Read the model definition and answer for the solid it produces. Units are mm, in the model's axes. Face numbers are marked on the shaded views. A direction names the side the tool comes from. Coordinates: 2 decimals unless noted, no trailing zeros. Write each loop counter-clockwise with the first axis right and the second up, starting at its lowest first coordinate (ties: lowest second). Pieces come first, ordered by that corner, then holes. Notation, with made-up numbers: (87, 68.25) -> (137, 68.25) arc R35 cw to (137, 103.25) -> close; hole circle Ø1 at (52.5, -21). An arc over 180 degrees is marked (long way). Answer in a Markdown table with one row per item. Add a question column.
Item 1: Section B-B on z = 0 is taken. Count the separate pieces of the cut face and the enclosed holes in it, then the cut area to 3 significant figures.
Item 2: Given pin 1 Ø6.5 at (y, z) = (-17.25, 0) entering from -X; pin 2 Ø5 at (x, y) = (-9, 2) entering from -Z; pin 3 Ø4 at (x, y) = (-1.5, -28) entering from +Z, each flat-ended and moving along its own axis, determine where each tip first touches the part or whether it passes through.
Item 3: For a pull along Y with two mould halves and no side action, classify the marked faces 3, 4 and 5 as +Y half, -Y half, draft (parallel to the pull), parting line (faces both ways), or undercut.
Item 4: Straight lines are drawn through the part: line 1 (Y direction, x = 1.5, z = 0); line 2 (Z direction, x = 8.5, y = -9); line 3 (X direction, y = 18, z = -2). For each, find the intervals that lie inside material, in ascending order. Write a range as from..to.
Item 5: Which of the six approach directions +Z, -Z, +X, -X, +Y, -Y give full straight-line access (tool end or side, diameter ignored) to the marked faces 1 and 2?
Item 6: Section A-A on x = 2.5 is taken. Write down the section's boundary in (y, z) (3 decimals).
```python
from build123d import *

# Parameters (mm, degrees)
SKETCH_1_R         = 28.5
SKETCH_1_R_2       = 1.9
SKETCH_1_R_3       = 7.5
EXTRUDE_1_DEPTH    = 10
SKETCH3_R          = 1.9
SKETCH3_R_2        = 7.5
CUT_EXTRUDE1_DEPTH = 60.270566179
SKETCH4_R          = 4
CUT_EXTRUDE2_DEPTH = 5


with BuildPart() as part:
    # 草图1 → 凸台-拉伸1 (new body)
    with BuildSketch(Plane(origin=(0, 0, 0), x_dir=(0, 0, -1), z_dir=(1, 0, 0))):
        Circle(SKETCH_1_R)
        with Locations((0, 17.25)):
            Circle(SKETCH_1_R_2, mode=Mode.SUBTRACT)
        with Locations((14.938938215, 8.625)):
            Circle(SKETCH_1_R_2, mode=Mode.SUBTRACT)
        with Locations((14.938938215, -8.625)):
            Circle(SKETCH_1_R_2, mode=Mode.SUBTRACT)
        with Locations((0, -17.25)):
            Circle(SKETCH_1_R_2, mode=Mode.SUBTRACT)
        with Locations((-14.938938215, -8.625)):
            Circle(SKETCH_1_R_2, mode=Mode.SUBTRACT)
        with Locations((-14.938938215, 8.625)):
            Circle(SKETCH_1_R_2, mode=Mode.SUBTRACT)
        Circle(SKETCH_1_R_3, mode=Mode.SUBTRACT)
    extrude(amount=EXTRUDE_1_DEPTH)

    # Sketch2 → Revolve1 (revolve)
    with BuildSketch(Plane.XY):
        with BuildLine():
            Line((0, 0), (-15, 0))
            Line((-15, 0), (-15, 38))
            Line((-15, 38), (-13, 38))
            add(Edge.make_bspline(
                [(-13, 38), (-9.977066976, 32.039576737), (-7.515495422, 32.019303811), (-5.003056497, 32.052880233), (-2, 38)],
                knots=[0.048051887, 0.048051887, 0.048051887, 0.048051887, 0.500504931, 0.951948113, 0.951948113, 0.951948113, 0.951948113], degree=3))
            Line((-2, 38), (0, 38))
            Line((0, 38), (0, 0))
        make_face()
    revolve(axis=Axis((0, 0, 0), (-1, 0, 0)))

    # Sketch3 → Cut-Extrude1 (cut, through all)
    with BuildSketch(Plane(origin=(10, 0, 0), x_dir=(0, 0, -1), z_dir=(1, 0, 0))):
        with Locations((14.938938215, 8.625)):
            Circle(SKETCH3_R)
        with Locations((14.938938215, -8.625)):
            Circle(SKETCH3_R)
        with Locations((0, -17.25)):
            Circle(SKETCH3_R)
        with Locations((-14.938938215, -8.625)):
            Circle(SKETCH3_R)
        with Locations((0, 17.25)):
            Circle(SKETCH3_R)
        with Locations((-14.938938215, 8.625)):
            Circle(SKETCH3_R)
        Circle(SKETCH3_R_2)
    extrude(amount=-CUT_EXTRUDE1_DEPTH, mode=Mode.SUBTRACT)

    # Sketch4 → Cut-Extrude2 (cut)
    with BuildSketch(Plane.ZY.offset(15)):
        with Locations(Location((14.938938215, 8.625, 0), (0, 0, 270))):
            Circle(SKETCH4_R)
        with Locations(Location((14.938938215, -8.625, 0), (0, 0, 270))):
            Circle(SKETCH4_R)
        with Locations(Location((0, -17.25, 0), (0, 0, 270))):
            Circle(SKETCH4_R)
        with Locations(Location((-14.938938215, -8.625, 0), (0, 0, 270))):
            Circle(SKETCH4_R)
        with Locations(Location((-14.938938215, 8.625, 0), (0, 0, 270))):
            Circle(SKETCH4_R)
        with Locations(Location((0, 17.25, 0), (0, 0, 270))):
            Circle(SKETCH4_R)
    extrude(amount=-CUT_EXTRUDE2_DEPTH, mode=Mode.SUBTRACT)


solid = part.part
```
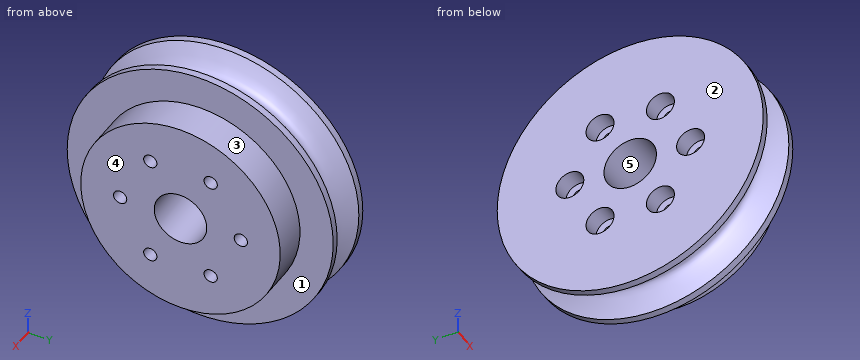
Results below:
| question | item | result |
|---|---|---|
| 1 | separate pieces | 4 |
| 1 | enclosed holes | 0 |
| 1 | area | 1,020 mm2 |
| 2 | pin 1 | stops at x = -10 |
| 2 | pin 2 | stops at z = -35.22 |
| 2 | pin 3 | stops at z = 27.71 |
| 3 | face 3 | parting line |
| 3 | face 4 | draft |
| 3 | face 5 | undercut |
| 4 | line 1 | y = -28.5..-19.15, -15.35..-7.5, 7.5..15.35, 19.15..28.5 |
| 4 | line 2 | z = -27.04..-16.8, -13.08..13.08, 16.8..27.04 |
| 4 | line 3 | x = -10..10 |
| 5 | face 1 | +X |
| 5 | face 2 | +Z, -Z, -X, +Y, -Y |
| 6 | outline | circle Ø57 at (0, 0); hole circle Ø3.8 at (-17.25, 0); hole circle Ø3.8 at (-8.625, -14.939); hole circle Ø3.8 at (-8.625, 14.939); hole circle Ø15 at (0, 0); hole circle Ø3.8 at (8.625, -14.939); hole circle Ø3.8 at (8.625, 14.939); hole circle Ø3.8 at (17.25, 0) |
